Verification items for the finished model (mm, model axes). A direction names the side the tool comes from. Give positions to 0.01 mm unless a question says otherwise; leave off trailing zeros. Write each loop counter-clockwise with the first axis right and the second up, starting at its lowest first coordinate (ties: lowest second). Pieces come first, ordered by that corner, then holes.
from build123d import *

# Parameters (mm, degrees)
F0_W     = 6.2
F0_H     = 3.35
F1_DEPTH = 1.8
F2_DEPTH = 9.8
F3_R     = 1


with BuildPart() as f1:
    # F0 (on Top) → F1 (new body)
    with BuildSketch(Plane.XY):
        with Locations((-4.898699, 1.675)):
            Rectangle(F0_W, F0_H)
        Polygon((-0.498699, 3.35), (-0.498699, 0), (6.001301, 0), (6.001301, 1.75), (4.001301, 3.35), align=None)
    extrude(amount=F1_DEPTH)

    # F0 (on Top) → F2 (join)
    with BuildSketch(Plane.XY):
        Polygon((-9.748699, 0), (-7.998699, 0), (-7.998699, 3.35), (-1.798699, 3.35), (-0.498699, 3.35), (4.001301, 3.35), (6.001301, 1.75), (6.001301, 0), (7.751301, 0), (7.751301, 2.591093), (4.615168, 5.1), (-9.748699, 5.1), align=None)
    extrude(amount=F2_DEPTH)

    # F3
    f3_edges = [f1.edges().sort_by_distance(p)[0] for p in [
        (-9.748699, 5.1, 4.9),
        (4.615168, 5.1, 4.9),
        (7.751301, 2.591093, 4.9),
        (-2.566765, 5.1, 0),
        (6.183235, 3.845547, 0),
        (7.751301, 1.295547, 0),
        (-9.748699, 2.55, 0),
    ]]
    fillet(f3_edges, radius=F3_R)

    # F4: F1 across face


with BuildPart() as f1_1:
    add(f1.part)
    add(f1.part.mirror(Plane(origin=(5.186004, 0, 3.300707), x_dir=(1, 0, 0), z_dir=(0, -1, 0))))


solid = f1_1.part
Item 1: Depth check by flat-ended pin: pin 1 (0.5 mm diameter, centred on y = -1, z = 0.5, fed in from +X); pin 2 (3 mm diameter, centred on x = 3.5, y = -1.5, fed in from +Z); pin 3 (1.5 mm diameter, centred on x = 5.5, z = 7, fed in from +Y). Enter the tip coordinate at first touch or a pass-through.
Answer key:
pin 1: stops at x = 7.72
pin 2: stops at z = 1.8
pin 3: stops at y = 4.97
Item 2: Scan lines: line 1 along Y through (x, z) = (-4.5, 3.5); line 2 along X through (y, z) = (0, 5.25); line 3 along X through (y, z) = (1, 1.25). Record each from-to range of solid material in increasing order.
Answer key:
line 1: y = -5.1 to -3.35, 3.35 to 5.1
line 2: x = -9.75 to -8, 6 to 7.75
line 3: x = -9.75 to -1.8, -0.5 to 7.75
Item 3: Sectioned sample at A-A on x = -1. Record the cut outline in (y, z).
Answer key:
outline: (-5.1, 1) arc R1 ccw to (-4.1, 0) - (-3.35, 0) - (-3.35, 9.8) - (-5.1, 9.8) - close; (3.35, 0) - (4.1, 0) arc R1 ccw to (5.1, 1) - (5.1, 9.8) - (3.35, 9.8) - close
Item 4: Sectioned sample at B-B on y = 1.5. Record the cut outline in (x, z), then the cut area to 3 significant figures.
Answer key:
outline: (-9.75, 1) arc R1 ccw to (-8.75, 0) - (-1.8, 0) - (-1.8, 1.8) - (-8, 1.8) - (-8, 9.8) - (-9.75, 9.8) - close; (-0.5, 0) - (6.75, 0) arc R1 ccw to (7.75, 1) - (7.75, 9.8) - (6, 9.8) - (6, 1.8) - (-0.5, 1.8) - close
area: 56.7 mm2
Item 5: Release check for a two-part mould opening along X. For faces 1 (the face through (-2.333, 4.799, 0.285)), 2 (the face through (-2, 3.35, 6)), 3 (the face through (7.451, -0.03, 0.285)) record: released by +X, released by -X, zero draft, split by the parting line, or undercut.
Answer key:
face 1: zero draft
face 2: undercut
face 3: released by +X
Item 6: Sectioned sample at D-D on x = 2. Record the cut outline in (y, z), then the cut area to 3 significant figures.
Answer key:
outline: (-5.1, 1) arc R1 ccw to (-4.1, 0) - (4.1, 0) arc R1 ccw to (5.1, 1) - (5.1, 9.8) - (3.35, 9.8) - (3.35, 1.8) - (-3.35, 1.8) - (-3.35, 9.8) - (-5.1, 9.8) - close
area: 45.9 mm2
Item 7: Sectioned sample at C-C on z = 2.25. Record the cut outline in (x, y), then the cut area to 3 significant figures.
Answer key:
outline: (-9.75, -4.1) arc R1 ccw to (-8.75, -5.1) - (4.26, -5.1) arc R1 ccw to (4.89, -4.88) - (7.38, -2.89) arc R1 ccw to (7.75, -2.11) - (7.75, 2.11) arc R1 ccw to (7.38, 2.89) - (4.89, 4.88) arc R1 ccw to (4.26, 5.1) - (-8.75, 5.1) arc R1 ccw to (-9.75, 4.1) - close; hole (-8, -3.35) - (4, -3.35) - (6, -1.75) - (6, 1.75) - (4, 3.35) - (-8, 3.35) - close
area: 79.5 mm2
Item 8: Set-up check for faces 4 (the face through (4.99, 2.56, 5.74)), 5 (the face through (6.15, -3.87, 5.34)), 6 (the face through (-0.499, 0, 1)): record each of +Z, -Z, +X, -X, +Y, -Y from which the full face is reachable in a straight line by a thin tool's end or side.
Answer key:
face 4: +Z
face 5: +Z, -Z, +X, -Y
face 6: +Z, -Z
